Read the model definition and answer for the solid it produces. Units are mm, in the model's axes. Face numbers are marked on the shaded views. A direction names the side the tool comes from. Give positions to 0.01 mm unless a question says otherwise; leave off trailing zeros. Order: outer loops, then holes, each group sorted by start corner. A loop starts at its lowest first (then second) coordinate and runs counter-clockwise, first axis right, second up. Notation, with made-up numbers: (52, 18.25) - (82, 18.25) arc R22 ccw to (82, 31.25) - close; hole circle Ø4 at (-16, 47). An arc over 180 degrees is marked (long way). Write each question's results on one line, items separated by ' | '. Start each with the question number.
Q1. Find section B-B on z = 1. Give the vertices of the cut face in (x, y) (3 decimals), and give its area (3 significant figures).
Q2. Find the intervals of material crossed by line 1 along Y through (x, z) = (6, -7.5); line 2 along X through (y, z) = (-30, -13.5) (3 decimals); line 3 along X through (y, z) = (-43, 10) (3 decimals), in increasing order. Write a range as from..to.
Q3. Find section C-C on x = -15.5. Give the vertices of the cut face in (y, z), and give its area (3 significant figures).
Q4. For a pull along X with two mould halves and no side action, classify the marked faces 5, 6, 7 and 8 as +X half, -X half, draft (parallel to the pull), parting line (faces both ways), or undercut.
Q5. A tool of negligible diameter and unlimited length cuts with its end or side. For the marked faces 1, 2, 3 and 4, from which of +Z, -Z, +X, -X, +Y, -Y can it reach the whole face along a straight path? Write none if from no direction.
Q6. Find section A-A on y = -37. Count the separate pieces of the cut face and the enclosed holes in it, and give its area (3 significant figures).
Q7. Find section D-D on z = 25.5. Give the vertices of the cut face in (x, y).
Q8. Flat-ended cylindrical pins translate along their axes: P1, Ø6, axis at x = 16, y = -41, coming from the -Z side; P2, Ø12, axis at x = -8.5, z = -10, coming from the -Y side; P3, Ø10, axis at x = -21.971, z = 0, coming from the -Y side; P4, Ø1, axis at y = -7.5, z = 0.5, coming from the +X side (3 decimals). Find the tip coordinate at first contact, or state that the pin passes through.
Autodesk Inventor part; units mm, degrees
ref_plane "YZ Plane" through (0, 0, 0) normal (1, 0, 0) x (0, 1, 0)
ref_plane "XZ Plane" through (0, 0, 0) normal (0, 1, 0) x (-1, 0, 0)
ref_plane "XY Plane" through (0, 0, 0) normal (0, 0, 1) x (1, 0, 0)
sketch "Sketch1" plane through (0, 0, 0) normal (0, 1, 0) x (-1, 0, 0)
  circle A0 centre (0, 0) radius 30.48
  line L0 (-6.35, 0) -> (-12.7, 6.35)
  line L1 (-12.7, 6.35) -> (-14.2875, 4.7625)
  line L2 (-14.2875, 4.7625) -> (-9.525, 0)
  line L3 (-9.525, 0) -> (-6.35, 0)
  line L4 (-6.35, 0) -> (-12.7, -6.35)
  line L5 (-12.7, -6.35) -> (-14.2875, -4.7625)
  line L6 (-14.2875, -4.7625) -> (-9.525, 0)
  line L7 (0, 30.48) -> (0, -30.48)
  line L8 (0, -6.35) -> (-6.35, -12.7)
  line L9 (-6.35, -12.7) -> (-4.7625, -14.2875)
  line L10 (-4.7625, -14.2875) -> (0, -9.525)
  line L11 (0, -9.525) -> (0, -6.35)
  line L12 (4.7625, -14.2875) -> (0, -9.525)
  line L13 (6.35, -12.7) -> (4.7625, -14.2875)
  line L14 (0, -6.35) -> (6.35, -12.7)
  line L15 (6.35, 0) -> (12.7, -6.35)
  line L16 (12.7, -6.35) -> (14.2875, -4.7625)
  line L17 (14.2875, -4.7625) -> (9.525, 0)
  line L18 (9.525, 0) -> (6.35, 0)
  line L19 (14.2875, 4.7625) -> (9.525, 0)
  line L20 (12.7, 6.35) -> (14.2875, 4.7625)
  line L21 (6.35, 0) -> (12.7, 6.35)
  line L22 (0, 6.35) -> (6.35, 12.7)
  line L23 (6.35, 12.7) -> (4.7625, 14.2875)
  line L24 (4.7625, 14.2875) -> (0, 9.525)
  line L25 (0, 9.525) -> (0, 6.35)
  line L26 (-4.7625, 14.2875) -> (0, 9.525)
  line L27 (-6.35, 12.7) -> (-4.7625, 14.2875)
  line L28 (0, 6.35) -> (-6.35, 12.7)
  circle A1 centre (21.971, 0) radius 3.81
  point P0 (-7.9375, 0)
  point P1 (0, -7.9375)
  point P2 (7.9375, 0)
  point P3 (0, 7.9375)
  dimension "d0" = 60.96
  dimension "d3" = 45
  dimension "d6" = 6.35
  dimension "d7" = 3.175
  dimension "d8" = 6.35
  dimension "d11" = 360
  dimension "d15" = 7.62
  dimension "d16" = 21.971
extrude "Extrusion1" add sketch "Sketch1" along normal blind 6.35 contours A0 L7 L12 L13 L14 L22 L23 L24 | L7 L26 L27 L28 L8 L9 L10 A0 | L24 L23 L22 L7 | L7 L28 L27 L26 | L10 L9 L8 L7 | L7 L14 L13 L12 | L3 L2 L1 L0 | L4 L5 L6 L3 | L18 L17 L16 L15 | L21 L20 L19 L18 | A1
extrude "Extrusion2" add sketch "Sketch1" against normal blind 50.8 contours L24 L23 L22 L7 | L7 L28 L27 L26 | L10 L9 L8 L7 | L7 L14 L13 L12 | L3 L2 L1 L0 | L4 L5 L6 L3 | L18 L17 L16 L15 | L21 L20 L19 L18
extrude "Extrusion3" cut sketch "Sketch1" along normal blind 6.35 contours A1
properties part number "OGPlatform" material "ABS Plastic"
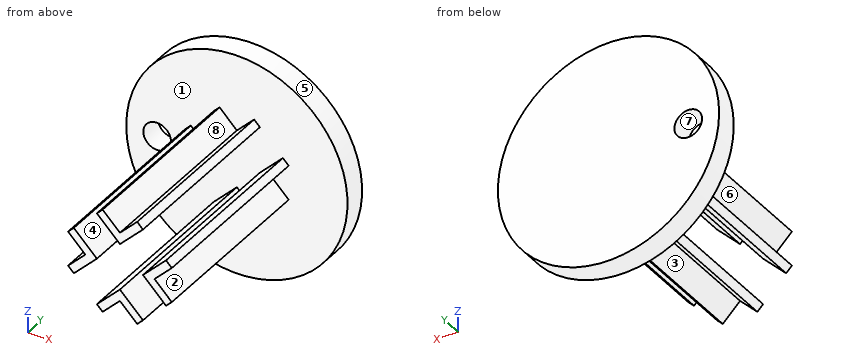
Working result:
1) outline: (-30.464, 0) - (-25.647, 0) - (-25.647, 6.35) - (-30.464, 6.35) - close; (-18.295, 0) - (-10.525, 0) - (-10.525, -50.8) - (-7.35, -50.8) - (-7.35, 0) - (7.35, 0) - (7.35, -50.8) - (10.525, -50.8) - (10.525, 0) - (30.464, 0) - (30.464, 6.35) - (-18.295, 6.35) - close | area: 663 mm²
2) line 1: 0..6.35 | line 2: -5.55..-3.975, 3.975..5.55 | line 3: -3.65..-0.475, 0.475..3.65
3) outline: (0, -26.24) - (6.35, -26.24) - (6.35, 26.24) - (0, 26.24) - close | area: 333 mm²
4) face 5: parting line | face 6: -X half | face 7: undercut | face 8: undercut
5) face 1: -Y | face 2: +X, -Y | face 3: -Z, -Y | face 4: +Z, -Y
6) separate pieces: 4 | enclosed holes: 0 | area: 141 mm²
7) outline: (-16.7, 0) - (16.7, 0) - (16.7, 6.35) - (-16.7, 6.35) - close
8) P1: z = -6.05 | P2: y = -50.8 | P3: y = 0 | P4: x = 10.525
